Autodesk Inventor part; units mm, degrees
ref_plane "YZ Plane" through (0, 0, 0) normal (1, 0, 0) x (0, 1, 0)
ref_plane "XZ Plane" through (0, 0, 0) normal (0, 1, 0) x (-1, 0, 0)
ref_plane "XY Plane" through (0, 0, 0) normal (0, 0, 1) x (1, 0, 0)
sketch "Sketch1" plane through (0, 0, 0) normal (0, 0, 1) x (1, 0, 0)
  line L0 (0, 0) -> (25.4, 0)
  line L1 (25.4, 0) -> (25.4, 3.175)
  line L2 (3.175, 50.8) -> (0, 50.8)
  line L3 (0, 50.8) -> (0, 0)
  line L4 (3.175, 50.8) -> (3.175, 3.175)
  line L5 (3.175, 3.175) -> (25.4, 3.175)
  dimension "d0" = 50.8
  dimension "d1" = 25.4
  dimension "d2" = 3.175
  dimension "d3" = 3.175
extrude "Extrusion1" add sketch "Sketch1" along normal blind 609.6
sketch "Sketch2" plane through (0, 0, 0) normal (-1, 0, 0) x (0, 0, 1)
  line L0 (609.6, 0) -> (609.6, 50.8)
  line L1 (0, 50.8) -> (609.6, 50.8)
  line L2 (0, 50.8) -> (0, 0)
  circle A0 centre (577.85, 31.75) radius 14.2875
  circle A1 centre (419.1, 31.75) radius 14.2875
  circle A2 centre (190.5, 31.75) radius 14.2875
  circle A3 centre (31.75, 31.75) radius 14.2875
  circle A4 centre (498.475, 31.75) radius 14.2875
  circle A5 centre (111.125, 31.75) radius 14.2875
  dimension "d6" = 28.575
  dimension "d7" = 31.75
  dimension "d8" = 19.05
  dimension "d9" = 28.575
  dimension "d10" = 228.6
  dimension "d11" = 31.75
  dimension "d15" = 158.75
  dimension "d16" = 79.375
  dimension "d17" = 79.375
  dimension "d18" = 609.6
extrude "Extrusion2" cut sketch "Sketch2" against normal through all
equation "\"d2\" = d3"
equation "\"d11\" = d7"
equation "\"d15\" = 0.5 * d18 - 0.5 * d10 - d7"
equation "\"d16\" = 0.5 * d15"
equation "\"d17\" = d16"
properties part number "maipulator L frame front"
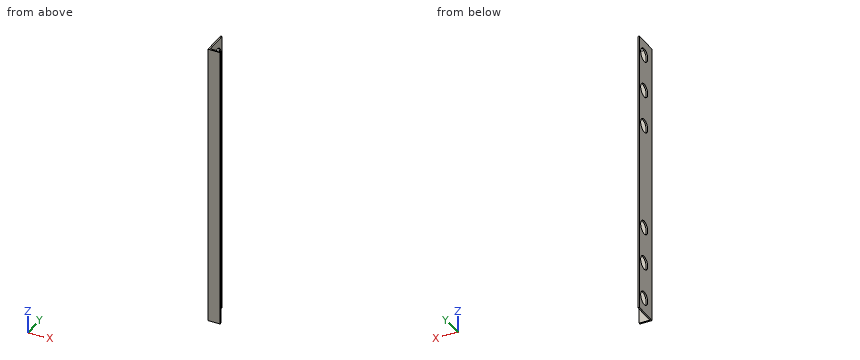
Geometry check sheet. Reference: the model listing, model coordinates, mm. Give positions to 0.01 mm unless a question says otherwise; leave off trailing zeros. Order: outer loops, then holes, each group sorted by start corner. A loop starts at its lowest first (then second) coordinate and runs counter-clockwise, first axis right, second up.
1) Cross-section at B-B (y = 31.75). Record the boundary of the cut face in (x, z) (1 decimal).
Results are:
outline: (0, 0) - (3.2, 0) - (3.2, 17.5) - (0, 17.5) - close; (0, 46) - (3.2, 46) - (3.2, 96.8) - (0, 96.8) - close; (0, 125.4) - (3.2, 125.4) - (3.2, 176.2) - (0, 176.2) - close; (0, 204.8) - (3.2, 204.8) - (3.2, 404.8) - (0, 404.8) - close; (0, 433.4) - (3.2, 433.4) - (3.2, 484.2) - (0, 484.2) - close; (0, 512.8) - (3.2, 512.8) - (3.2, 563.6) - (0, 563.6) - close; (0, 592.1) - (3.2, 592.1) - (3.2, 609.6) - (0, 609.6) - close
2) Cross-section at A-A (z = 577.85). Record the boundary of the cut face in (x, y) (1 decimal).
Results are:
outline: (0, 0) - (25.4, 0) - (25.4, 3.2) - (3.2, 3.2) - (3.2, 17.5) - (0, 17.5) - close; (0, 46) - (3.2, 46) - (3.2, 50.8) - (0, 50.8) - close
3) Cross-section at D-D (z = 193). Record the boundary of the cut face in (x, y) (3 decimals), then the cut area to 3 significant figures.
Results are:
outline: (0, 0) - (25.4, 0) - (25.4, 3.175) - (3.175, 3.175) - (3.175, 17.683) - (0, 17.683) - close; (0, 45.817) - (3.175, 45.817) - (3.175, 50.8) - (0, 50.8) - close
area: 143 mm2
4) Cross-section at C-C (x = 9.75). Record the boundary of the cut face in (y, z) (3 decimals), then the cut area to 3 significant figures.
Results are:
outline: (0, 0) - (3.175, 0) - (3.175, 609.6) - (0, 609.6) - close
area: 1,940 mm2
5) Material ranges on probe 1 along Y at (x, z) = (2.35, 419.1); probe 2 along X at (y, z) = (17, 25) (3 decimals), recorded low to high.
Results are:
probe 1: y = 0 to 17.46, 46.04 to 50.8
probe 2: x = 0 to 3.175
6) Gauge pin test, flat ends, axial feed: pin 1 (12 mm diameter, centred on x = 4, z = 354.5, fed in from -Y); pin 2 (5 mm diameter, centred on y = 41.5, z = 149, fed in from +X) (3 decimals); pin 3 (23 mm diameter, centred on y = 31.75, z = 419.1, fed in from +X); pin 4 (2 mm diameter, centred on x = 7, z = 363, fed in from +Y) (3 decimals). Record the tip position at first contact, or that the pin passes through.
Results are:
pin 1: stops at y = 0
pin 2: stops at x = 3.175
pin 3: passes through
pin 4: stops at y = 3.175
